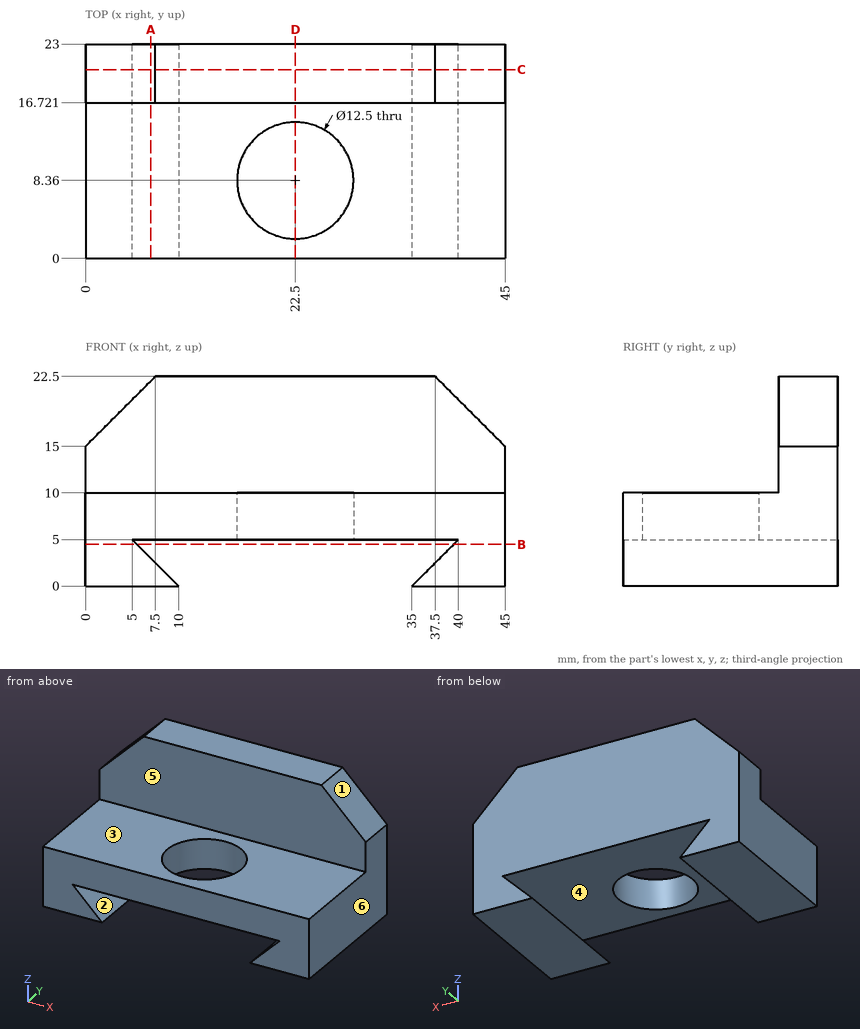
Geometry check sheet. Reference: drawing and pictorial views, mm from the part's lowest x, y, z. A direction names the side the tool comes from. Round coordinates to 2 decimals unless told otherwise and drop trailing zeros. Loops run counter-clockwise (first coordinate to the right, second up) from the corner with the lowest first, then second, coordinate; pieces in that order, holes last. Notation, with made-up numbers: (30, 84.25) -> (46, 84.25) arc R31 cw to (46, 111.25) -> close; hole circle Ø7 at (82.5, -19). An arc over 180 degrees is marked (long way). Answer as a JSON object with one key per item and string values. Group by question number.
Item 1: Release check for a two-part mould opening along X. For the marked faces 1, 2 and 3 record: pulls with the +X half, pulls with the -X half, needs draft (parallel to the pull), parting line crosses it, or undercut.
Item 2: Cross-section at C-C, the plane y = 20.25. Record the cut outline in (x, z), plus the area to 3 significant figures.
Item 3: Thickness scan on line 1 along Y through (x, z) = (22.5, 6.1); line 2 along X through (y, z) = (8.5, 9); line 3 along Z through (x, y) = (9, 1). Record the ranges inside material, lowest first.
Item 4: Depth check by flat-ended pin: pin 1 Ø6 at (x, z) = (17, 13.5) entering from -Y; pin 2 Ø8.5 at (x, y) = (28, 7) entering from +Z; pin 3 Ø2 at (x, y) = (26.5, 20) entering from -Z. Enter the tip coordinate at first touch or a pass-through.
Item 5: Cross-section at D-D, the plane x = 22.5. Record the cut outline in (y, z), plus the area to 3 significant figures.
Item 6: Cross-section at B-B, the plane z = 4.5. Record the cut outline in (x, y), plus the area to 3 significant figures.
Item 7: Cross-section at A-A, the plane x = 7. Record the cut outline in (y, z).
Item 8: Set-up check for the marked faces 4, 5 and 6: record each of +Z, -Z, +X, -X, +Y, -Y from which the full face is reachable in a straight line by a thin tool's end or side.
Determined:
{
 "1": {"face 1": "pulls with the +X half", "face 2": "undercut", "face 3": "needs draft"},
 "2": {"outline": "(0, 0) -> (10, 0) -> (5, 5) -> (40, 5) -> (35, 0) -> (45, 0) -> (45, 15) -> (37.5, 22.5) -> (7.5, 22.5) -> (0, 15) -> close", "area": "806 mm²"},
 "3": {"line 1": "y = 0 to 2.11, 14.61 to 23", "line 2": "x = 0 to 16.25, 28.75 to 45", "line 3": "z = 0 to 1, 5 to 10"},
 "4": {"pin 1": "stops at y = 16.72", "pin 2": "stops at z = 10", "pin 3": "stops at z = 5"},
 "5": {"outline": "(0, 5) -> (2.11, 5) -> (2.11, 10) -> (0, 10) -> close; (14.61, 5) -> (23, 5) -> (23, 22.5) -> (16.72, 22.5) -> (16.72, 10) -> (14.61, 10) -> close", "area": "131 mm²"},
 "6": {"outline": "(0, 0) -> (5.5, 0) -> (5.5, 23) -> (0, 23) -> close; (39.5, 0) -> (45, 0) -> (45, 23) -> (39.5, 23) -> close", "area": "253 mm²"},
 "7": {"outline": "(0, 0) -> (23, 0) -> (23, 3) -> (0, 3) -> close; (0, 5) -> (23, 5) -> (23, 22) -> (16.72, 22) -> (16.72, 10) -> (0, 10) -> close"},
 "8": {"face 4": "+Y, -Y", "face 5": "+Z, +X, -X, -Y", "face 6": "+Z, -Z, +X, +Y, -Y"}
}
